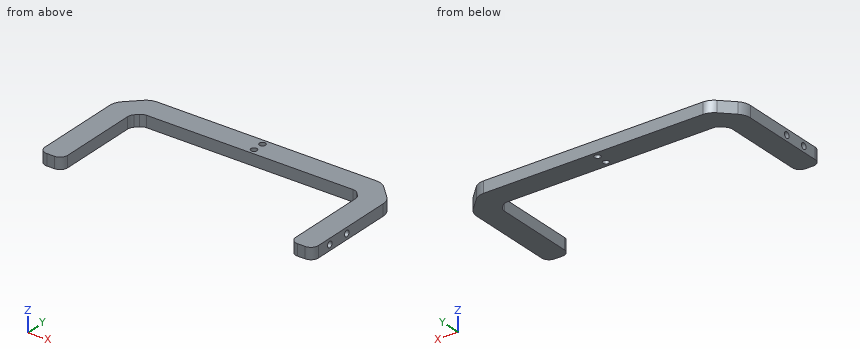
from build123d import *

# Parameters (mm, degrees)
BOSS_EXTRUDE1_DEPTH              = 9.525
FILLET3_R                        = 6.35
FILLET1_R                        = 12.7
F_1_4_20_TAPPED_HOLE1_D          = 5.1054
F_1_4_20_TAPPED_HOLE2_AT_2_COUNT = 2
F_1_4_20_TAPPED_HOLE2_AT_2_PITCH = 19.05


with BuildPart() as part:
    # Sketch1 → Boss-Extrude1 (new body)
    with BuildSketch(Plane.XY):
        Polygon((-114.3, -17.509231637), (-96.790768363, 0), (96.790768363, 0), (114.3, -17.509231637), (114.3, -101.6), (95.25, -101.6), (95.25, -25.4), (88.9, -19.05), (-88.9, -19.05), (-95.25, -25.4), (-95.25, -101.6), (-114.3, -101.6), align=None)
    extrude(amount=BOSS_EXTRUDE1_DEPTH)

    # Fillet3
    fillet3_edges = [part.edges().sort_by_distance(p)[0] for p in [
        (114.3, -101.6, 4.7625),
        (95.25, -101.6, 4.7625),
        (95.25, -25.4, 4.7625),
        (88.9, -19.05, 4.7625),
        (-88.9, -19.05, 4.7625),
        (-95.25, -25.4, 4.7625),
        (-95.25, -101.6, 4.7625),
        (-114.3, -101.6, 4.7625),
    ]]
    fillet(fillet3_edges, radius=FILLET3_R)

    # Fillet1
    fillet1_edges = [part.edges().sort_by_distance(p)[0] for p in [
        (-114.3, -17.509231637, 4.7625),
        (-96.790768363, 0, 4.7625),
        (96.790768363, 0, 4.7625),
        (114.3, -17.509231637, 4.7625),
    ]]
    fillet(fillet1_edges, radius=FILLET1_R)

    # 1/4-20 Tapped Hole1 (through all)
    with Locations(Plane.XY.offset(9.525)):
        with Locations((0, -4.7625), (0, -14.2875)):
            Hole(F_1_4_20_TAPPED_HOLE1_D / 2)

    # Sketch5 → 1/4-20 Tapped Hole2 (revolve, cut)
    with BuildSketch(Plane(origin=(114.3, -82.55, 4.7625), x_dir=(0, 0, -1), z_dir=(0, 1, 0))):
        Polygon((0, 0), (0, 17.408816902), (2.5527, 15.875), (2.5527, 0), align=None)
    f_1_4_20_tapped_hole2 = revolve(axis=Axis((120.65, -82.55, 4.7625), (-1, 0, 0)), mode=Mode.SUBTRACT)

    # 1/4-20 Tapped Hole2 at 2: 1/4-20 Tapped Hole2 ×2
    with Locations(*[(0, i * F_1_4_20_TAPPED_HOLE2_AT_2_PITCH, 0) for i in range(1, F_1_4_20_TAPPED_HOLE2_AT_2_COUNT)]):
        add(f_1_4_20_tapped_hole2, mode=Mode.SUBTRACT)

    # Mirror1: 1/4-20 Tapped Hole2 across plane
    add(f_1_4_20_tapped_hole2.mirror(Plane(origin=(0, 0, 0), x_dir=(0, 0, 1), z_dir=(1, 0, 0))), mode=Mode.SUBTRACT)

    # Mirror1 copy 1 sketch → Mirror1 copy 1 (revolve, cut)
    with BuildSketch(Plane(origin=(-114.3, -63.5, 4.7625), x_dir=(0, 0, -1), z_dir=(0, 1, 0))):
        Polygon((0, 0), (0, -17.408816902), (2.5527, -15.875), (2.5527, 0), align=None)
    revolve(axis=Axis((-120.65, -63.5, 4.7625), (-1, 0, 0)), mode=Mode.SUBTRACT)


solid = part.part
The model under review builds one solid part; all positions refer to its coordinate system, in mm. Round coordinates to 2 decimals unless told otherwise and drop trailing zeros. Write each loop counter-clockwise with the first axis right and the second up, starting at its lowest first coordinate (ties: lowest second). Pieces come first, ordered by that corner, then holes. Notation, with made-up numbers: M 81,5 L 116,5 A16 ccw 116,26 Z; hole C -34.5,46 d9. An arc over 180 degrees is marked long. Answer as CSV lines item,"result". Start each with the question number.
Q1. Clearance check with flat-ended pins moving along their axes: P1, Ø4, axis at y = -82.55, z = 4.76, coming from the +X side; P2, Ø5, axis at x = 36, z = 7.5, coming from the -Y side. State where each tip first meets the part, or that it passes through.
Q2. Consider section B-B, the plane x = 0. Give the boundary of the cut face in (y, z) (3 decimals), then the cut area to 3 significant figures.
Q3. Consider section C-C, the plane x = -39. Give the boundary of the cut face in (y, z) (3 decimals).
Q4. Consider section A-A, the plane y = -39.5. Give the boundary of the cut face in (x, z) (3 decimals), then the cut area to 3 significant figures.
Q5. Wall thickness on line 1 along Y through (x, z) = (0, 6); line 2 along X through (y, z) = (-28, 1); line 3 along Z through (x, y) = (103, -63) (3 decimals): over which ranges is each line inside the solid? List them lowest first.
Result set:
1,P1,"stops at x = 98.09"
1,P2,"stops at y = -19.05"
2,outline,"M -19.05,0 L -16.84,0 L -16.84,9.525 L -19.05,9.525 Z; M -11.735,0 L -7.315,0 L -7.315,9.525 L -11.735,9.525 Z; M -2.21,0 L 0,0 L 0,9.525 L -2.21,9.525 Z"
2,area,"84.2 mm²"
3,outline,"M -19.05,0 L 0,0 L 0,9.525 L -19.05,9.525 Z"
4,outline,"M -114.3,0 L -95.25,0 L -95.25,9.525 L -114.3,9.525 Z; M 95.25,0 L 114.3,0 L 114.3,9.525 L 95.25,9.525 Z"
4,area,"363 mm²"
5,line 1,"y = -19.05 to -16.84, -11.73 to -7.32, -2.21 to 0"
5,line 2,"x = -114.3 to -95.25, 95.25 to 114.3"
5,line 3,"z = 0 to 2.259, 7.266 to 9.525"
